```python
from build123d import *

# Parameters (mm, degrees)
MAIN_DEPTH                  = 100
FIXFORROLLINGCYLINDER_DEPTH = 5
SKETCH4_W                   = 10
SKETCH4_H                   = 10
HORIZONTALCUT_DEPTH         = 10
SKETCH7_W                   = 10
SKETCH7_H                   = 10
BOSS_EXTRUDE1_DEPTH         = 1
MAKERBEAMHOLE_DEPTH         = 101.931998276
MAKERBEAMHOLE_DEPTH_BACK    = 101.931998276
SKETCH5_R                   = 1.6
FILLET1_R                   = 10
FILLET2_R                   = 5
FILLET3_R                   = 0.5


with BuildPart() as part:
    # Sketch1 → Main (new body)
    with BuildSketch(Plane.XY):
        with BuildLine():
            Line((0, 0), (3.55, 0))
            Line((3.55, 0), (3.55, -1))
            Line((3.55, -1), (6.45, -1))
            Line((6.45, -1), (6.45, 0))
            Line((6.45, 0), (10, 0))
            Line((10, 0), (10, 8))
            Line((10, 8), (7.562177826, 8))
            Line((7.562177826, 8), (5.397114317, 4.25))
            ThreePointArc((5.397114317, 4.25), (3.75, 2.602885683), (1.5, 2))
            Line((1.5, 2), (0, 2))
            Line((0, 2), (0, 0))
        make_face()
    extrude(amount=MAIN_DEPTH)

    # Sketch3 → FixForRollingCylinder (add)
    with BuildSketch(Plane.XY.offset(90)):
        with BuildLine():
            Line((-1.50520382, 5.616116524), (0, 4.110912703))
            Line((0, 4.110912703), (0, 0))
            Line((0, 0), (10, 0))
            Line((10, 0), (10, 8))
            Line((10, 8), (7.562177826, 8))
            Line((7.562177826, 8), (4.220428741, 11.341749085))
            Line((4.220428741, 11.341749085), (1.323223305, 8.444543648))
            Line((1.323223305, 8.444543648), (2.383883476, 7.383883476))
            ThreePointArc((2.383883476, 7.383883476), (2.383883476, 5.616116524), (0.616116524, 5.616116524))
            Line((0.616116524, 5.616116524), (-0.444543648, 6.676776695))
            Line((-0.444543648, 6.676776695), (-1.50520382, 5.616116524))
        make_face()
    extrude(amount=-FIXFORROLLINGCYLINDER_DEPTH)

    # Sketch4 → HorizontalCut (cut)
    with BuildSketch(Plane(origin=(0, 3, 0), x_dir=(1, 0, 0), z_dir=(0, 1, 0))):
        with Locations((5, -95)):
            Rectangle(SKETCH4_W, SKETCH4_H)
    extrude(amount=HORIZONTALCUT_DEPTH, mode=Mode.SUBTRACT)

    # Sketch7 → Boss-Extrude1 (add)
    with BuildSketch(Plane(origin=(0, 3, 0), x_dir=(1, 0, 0), z_dir=(0, 1, 0))):
        with Locations((5, -95)):
            Rectangle(SKETCH7_W, SKETCH7_H)
    extrude(amount=-BOSS_EXTRUDE1_DEPTH)

    # Sketch5 → MakerBeamHole (cut, two sides: drawn at the far end of the back side and taken through both)
    with BuildSketch(Plane(origin=(0, 2, 0), x_dir=(1, 0, 0), z_dir=(0, 1, 0)).offset(-MAKERBEAMHOLE_DEPTH_BACK)):
        with Locations(Location((5, -95, 0), (0, 0, 25.007833235))):
            Circle(SKETCH5_R)
    extrude(amount=MAKERBEAMHOLE_DEPTH + MAKERBEAMHOLE_DEPTH_BACK, mode=Mode.SUBTRACT)

    # Mirror1: part across plane


with BuildPart() as part_1:
    add(part.part)
    add(part.part.mirror(Plane.XY))

    # Fillet1
    # the kernel refuses this fillet: 10 mm, written as the material it adds along each edge
    with BuildSketch(Plane(origin=(7.562177826, 8, -90), x_dir=(-0.7071067811865462, 0.7071067811865489, 0), z_dir=(0, 0, 1))) as fillet1_piece_1:
        with BuildLine():
            CenterArc((3.889088446, -10), FILLET1_R, 90, 34.144980958)
            Line((-1.72380059, -1.72380059), (0, 0))
            Line((0, 0), (3.889088446, 0))
        make_face()
    extrude(amount=5)
    with BuildSketch(Plane(origin=(7.562177826, 8, 90), x_dir=(-0.7071067811865462, 0.7071067811865489, 0), z_dir=(0, 0, -1))) as fillet1_piece_2:
        with BuildLine():
            CenterArc((3.889088446, 10), FILLET1_R, 235.855019042, 34.144980958)
            Line((-1.72380059, 1.72380059), (0, 0))
            Line((0, 0), (3.889088446, 0))
        make_face()
    extrude(amount=5)

    # Fillet2
    # the kernel refuses this fillet: 5 mm, written as the material it takes off along each edge
    with BuildSketch(Plane(origin=(4.220428741, 11.341749085, -100.243168054), x_dir=(0.7792084739241206, -0.6267648316273362, 0), z_dir=(0, 0, 1))) as fillet2_piece_1:
        with BuildLine():
            CenterArc((4.485150557, -4.925762162), FILLET2_R, 99.885624433, 70.299011634)
            Line((-0.441660549, -4.073393505), (-0.93434166, -3.988156639))
            ThreePointArc((-0.93434166, -3.988156639), (-0.717916904, -1.982799786), (-0.497086629, 0.053896967))
            Line((-0.497086629, 0.053896967), (0.053896967, 0.497086629))
            ThreePointArc((0.053896967, 0.497086629), (0.885879241, 0.406878367), (3.540899942, 0.492576216))
            Line((3.540899942, 0.492576216), (3.626740907, 0))
        make_face()
    extrude(amount=25.486336108, mode=Mode.SUBTRACT)
    with BuildSketch(Plane(origin=(4.220428741, 11.341749085, 100.243168054), x_dir=(0.7792084739241207, -0.626764831627336, 0), z_dir=(0, 0, -1))) as fillet2_piece_2:
        with BuildLine():
            CenterArc((4.485150557, 4.925762162), FILLET2_R, 189.815363933, 70.299011634)
            Line((-0.441660549, 4.073393505), (-0.93434166, 3.988156639))
            ThreePointArc((-0.93434166, 3.988156639), (-0.717916904, 1.982799786), (-0.497086629, -0.053896967))
            Line((-0.497086629, -0.053896967), (0.053896967, -0.497086629))
            ThreePointArc((0.053896967, -0.497086629), (0.885879241, -0.406878367), (3.540899942, -0.492576216))
            Line((3.540899942, -0.492576216), (3.626740907, 0))
        make_face()
    extrude(amount=25.486336108, mode=Mode.SUBTRACT)

    # Fillet3
    fillet3_edges = [part_1.edges().sort_by_distance(p)[0] for p in [
        (-1.50520382, 5.616116524, -87.5),
        (-1.50520382, 5.616116524, 87.5),
    ]]
    fillet(fillet3_edges, radius=FILLET3_R)


solid = part_1.part
```
The model under review builds one solid part; all positions refer to its coordinate system, in mm. A direction names the side the tool comes from. Round coordinates to 2 decimals unless told otherwise and drop trailing zeros. Loops run counter-clockwise (first coordinate to the right, second up) from the corner with the lowest first, then second, coordinate; pieces in that order, holes last. Notation, with made-up numbers: (-0.75, 15.25) -> (58.25, 15.25) arc R19 cw to (58.25, 36.25) -> close; hole circle Ø9 at (52, 66). An arc over 180 degrees is marked (long way). Answer as a JSON object with one key per item and string values. Group by question number.
1) We need section A-A on z = 12.5. Write out the cut boundary in (x, y), then the cut area to 3 significant figures.
2) Mouldability with a two-part tool opening along Z and no side actions: class faces 1 (the face through (5, 3, -93)), 2 (the face through (5, 1, 100)), 3 (the face through (4, 6, 85)), 4 (the face through (5, 1, -100)) as released by +Z, released by -Z, zero draft, split by the parting line, or undercut.
3) For pin 1 Ø1.2 at (x, z) = (9, 37.5) entering from +Y; pin 2 Ø1.8 at (x, z) = (2, -50) entering from -Y; pin 3 Ø4 at (x, z) = (5, 95) entering from -Y; pin 4 Ø5.5 at (x, y) = (2.5, 6) entering from +Z, all flat-tipped, find the tip position at first contact; note any pin that passes through.
4) For line 1 (Z direction, x = 5, y = 0); line 2 (X direction, y = 1.1, z = 95); line 3 (Z direction, x = 5.25, y = 6.5), list the stretches that pass through material, from the lowest coordinate up. Write a range as [from, to].
5) For faces 5 (the face through (4, 6, -85)), 6 (the face through (0, 1, -1)), 7 (the face through (5, 5, 90)), 8 (the face through (8, 0, 1)), list the 3-axis set-ups (+Z, -Z, +X, -X, +Y, -Y) from which the entire face can be reached by the end or side of a thin tool; tool diameter is ignored.
Result set:
{
 "1": {"outline": "(0, 0) -> (3.55, 0) -> (3.55, -1) -> (6.45, -1) -> (6.45, 0) -> (10, 0) -> (10, 8) -> (7.56, 8) -> (5.4, 4.25) arc R4.5 cw to (1.5, 2) -> (0, 2) -> close", "area": "49.0 mm²"},
 "2": {"face 1": "zero draft", "face 2": "released by +Z", "face 3": "undercut", "face 4": "released by -Z"},
 "3": {"pin 1": "y = 8", "pin 2": "y = 0", "pin 3": "y = -1", "pin 4": "z = 90"},
 "4": {"line 1": "[-100, -96.6], [-93.4, 93.4], [96.6, 100]", "line 2": "[0, 3.4], [6.6, 10]", "line 3": "[-90, -85], [85, 90]"},
 "5": {"face 5": "-X, +Y", "face 6": "+Z, -Z, -X, -Y", "face 7": "+Z, +X, -X, +Y", "face 8": "+Z, -Z, +X, -Y"}
}
